Model file for the job. Use its own axes, mm. A direction names the side the tool comes from. Give positions to 0.01 mm unless a question says otherwise; leave off trailing zeros. Loops run counter-clockwise (first coordinate to the right, second up) from the corner with the lowest first, then second, coordinate; pieces in that order, holes last. Notation, with made-up numbers: M 30,-2.5 L 61,-2.5 A17 cw 61,19.5 Z; hole C -15.5,61 d9. An arc over 180 degrees is marked long. Answer in a Markdown table with one row per item.
```python
from build123d import *

# Parameters (mm, degrees)
F0_W     = 2000
F0_H     = 500
F0_W_2   = 1860
F0_H_2   = 360
F1_DEPTH = 70
F2_W     = 30
F2_H     = 360
F3_DEPTH = 25
F4_DEPTH = 25
F5_W     = 360
F5_H     = 30
F6_DEPTH = 25
F7_SCALE = 0.4


with BuildPart() as f1:
    # F0 (on Front) → F1 (new body)
    with BuildSketch(Plane.XZ):
        with Locations((18.9460813999, -353.4244084814)):
            Rectangle(F0_W, F0_H)
        with Locations((18.9460813999, -353.4244084814)):
            Rectangle(F0_W_2, F0_H_2, mode=Mode.SUBTRACT)
    extrude(amount=F1_DEPTH)



with BuildPart() as f3:
    # F2 (on face) → F3 (new body)
    with BuildSketch(Plane(origin=(0, 0, 0), x_dir=(-1, 0, 0), z_dir=(0, 1, 0))):
        with Locations((946.0539186001, -353.4244084814)):
            Rectangle(F2_W, F2_H)
    extrude(amount=-F3_DEPTH)


with BuildPart() as f1_1:
    add(f1.part)

    add(f3.part)  # F4 merges F3
    # F2 (on face) → F4 (join)
    with BuildSketch(Plane(origin=(0, 0, 0), x_dir=(-1, 0, 0), z_dir=(0, 1, 0))):
        with Locations((-983.9460813999, -353.4244084814)):
            Rectangle(F2_W, F2_H)
        with Locations((946.0539186001, -353.4244084814)):
            Rectangle(F2_W, F2_H)
    extrude(amount=F4_DEPTH)

    # F5 (on face) → F6 (cut)
    with BuildSketch(Plane.XY.offset(-103.4244084814)):
        with Locations((-601.0539186001, -35)):
            Rectangle(F5_W, F5_H)
    extrude(amount=-F6_DEPTH, mode=Mode.SUBTRACT)


with BuildPart() as f1_2:
    # F7: moved
    add(f1_1.part.scale(F7_SCALE).moved(Location((611.36764884, -42, -362.0546450888))))


solid = f1_2.part
```
(1) Saw through at B-B, the plane x = 866.5. Give the cut face in (y, z), and give its area (3 significant figures).
Established:
| item | result |
|---|---|
| outline | M -70,-603.42 L -42,-603.42 L -42,-575.42 L -70,-575.42 Z; M -70,-431.42 L -42,-431.42 L -42,-403.42 L -70,-403.42 Z |
| area | 1,570 mm2 |
(2) Saw through at A-A, the plane z = -468. Give the cut face in (x, y), and give its area (3 significant figures).
Established:
| item | result |
|---|---|
| outline | M 218.95,-70 L 246.95,-70 L 246.95,-42 L 238.95,-42 L 238.95,-32 L 226.95,-32 L 226.95,-42 L 218.95,-42 Z; M 990.95,-70 L 1018.95,-70 L 1018.95,-42 L 1010.95,-42 L 1010.95,-32 L 998.95,-32 L 998.95,-42 L 990.95,-42 Z |
| area | 1,810 mm2 |
(3) Which spindle directions (+Z, -Z, +X, -X, +Y, -Y) get a long thin tool onto all of the face, cutting with end or side? Do faces 5 (the flat face through (1018.946, -56, -505)), 6 (the flat face through (246.946, -56, -504)). Say none if no direction does.
Established:
| item | result |
|---|---|
| face 5 | +Z, -Z, +X, +Y, -Y |
| face 6 | +Y, -Y |
(4) Mould opens along X. For faces 1 (the flat face through (990.946, -56, -504)), 2 (the flat face through (614, -56, -575.424)), 3 (the flat face through (613, -56, -403.424)), 4 (the flat face through (218.946, -56, -505)) say: pulls with the +X half, pulls with the -X half, needs draft (parallel to the pull), parting line crosses it, or undercut.
Established:
| item | result |
|---|---|
| face 1 | undercut |
| face 2 | undercut |
| face 3 | needs draft |
| face 4 | pulls with the -X half |
(5) Flat gauge pins, fed straight in: P1, Ø12, axis at x = 531, z = -574.5, coming from the -Y side; P2, Ø3, axis at x = 387, z = -409.5, coming from the +Y side; P3, Ø3, axis at y = -39.5, z = -501.5, coming from the -X side; P4, Ø6, axis at x = 356, y = -55.5, coming from the +Z side. Where does each tip first touch, or does it go through?
Established:
| item | result |
|---|---|
| P1 | stops at y = -70 |
| P2 | stops at y = -42 |
| P3 | stops at x = 226.95 |
| P4 | stops at z = -413.42 |
(6) Saw through at C-C, the plane x = 343.5. Give the cut face in (y, z), and give its area (3 significant figures).
Established:
| item | result |
|---|---|
| outline | M -70,-603.42 L -42,-603.42 L -42,-575.42 L -70,-575.42 Z; M -70,-431.42 L -42,-431.42 L -42,-403.42 L -50,-403.42 L -50,-413.42 L -62,-413.42 L -62,-403.42 L -70,-403.42 Z |
| area | 1,450 mm2 |
(7) Wall check: L1, parallel to X at y = -59.5, z = -527; L2, parallel to X at y = -35, z = -489.5; L3, parallel to Z at x = 621, y = -42.5. Give the ranges that are in metal, low to high.
Established:
| item | result |
|---|---|
| L1 | x = 218.95 to 246.95, 990.95 to 1018.95 |
| L2 | x = 226.95 to 238.95, 998.95 to 1010.95 |
| L3 | z = -603.42 to -575.42, -431.42 to -403.42 |
